Print and shaded views of the part. All mm, measured from the part's lowest x, y and z. A direction names the side the tool comes from. Round coordinates to 2 decimals unless told otherwise and drop trailing zeros. Write each loop counter-clockwise with the first axis right and the second up, starting at its lowest first coordinate (ties: lowest second). Pieces come first, ordered by that corner, then holes.
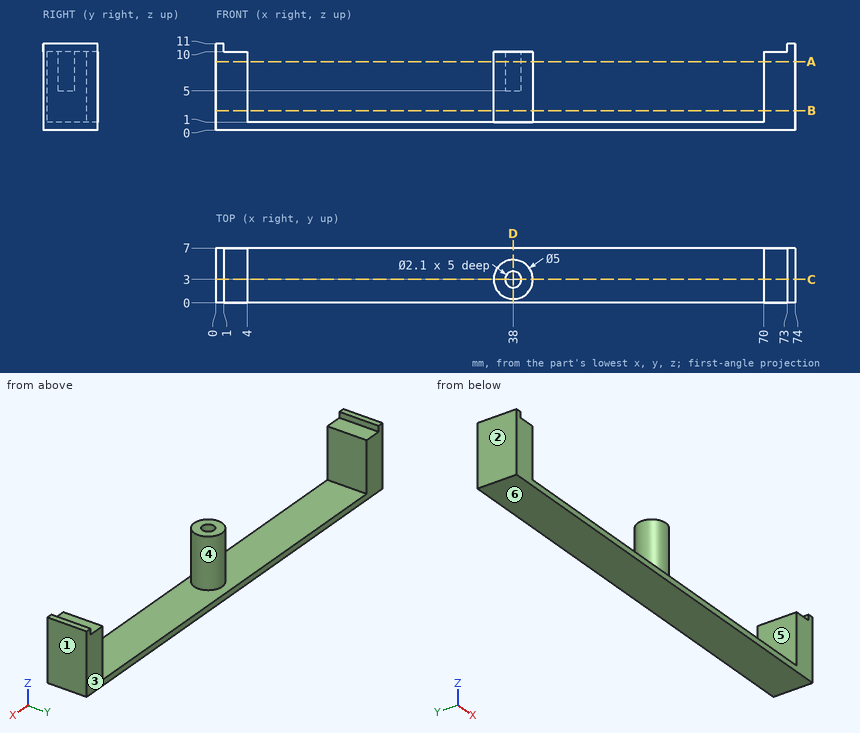
1) Slice it at A-A (z = 8.75). Write the cut outline in (x, y), plus the area to 3 significant figures.
Results:
outline: (0, 0) - (4, 0) - (4, 7) - (0, 7) - close; circle Ø5 at (38, 3); (70, 0) - (74, 0) - (74, 7) - (70, 7) - close; hole circle Ø2.1 at (38, 3)
area: 72.2 mm2
2) Slice it at C-C (y = 3). Write the cut outline in (x, z).
Results:
outline: (0, 0) - (74, 0) - (74, 11) - (73, 11) - (73, 10) - (70, 10) - (70, 1) - (40.5, 1) - (40.5, 10) - (39.05, 10) - (39.05, 5) - (36.95, 5) - (36.95, 10) - (35.5, 10) - (35.5, 1) - (4, 1) - (4, 10) - (1, 10) - (1, 11) - (0, 11) - close
3) Wall check: L1, parallel to X at y = 3, z = 8.25; L2, parallel to X at y = 6.5, z = 3.75; L3, parallel to X at y = 6.5, z = 10.5. Give the ranges that are in metal, low to high.
Results:
L1: x = 0 to 4, 35.5 to 36.95, 39.05 to 40.5, 70 to 74
L2: x = 0 to 4, 70 to 74
L3: x = 0 to 1, 73 to 74
4) Which spindle directions (+Z, -Z, +X, -X, +Y, -Y) get a long thin tool onto all of the face, cutting with end or side? Do the marked faces 5 and 6. Say none if no direction does.
Results:
face 5: +Z, +Y, -Y
face 6: -Z, +X, -X, +Y, -Y
5) Slice it at D-D (x = 38). Write the cut outline in (y, z).
Results:
outline: (0, 0) - (7, 0) - (7, 1) - (5.5, 1) - (5.5, 10) - (4.05, 10) - (4.05, 5) - (1.95, 5) - (1.95, 10) - (0.5, 10) - (0.5, 1) - (0, 1) - close
6) Slice it at B-B (z = 2.5). Write the cut outline in (x, y).
Results:
outline: (0, 0) - (4, 0) - (4, 7) - (0, 7) - close; circle Ø5 at (38, 3); (70, 0) - (74, 0) - (74, 7) - (70, 7) - close
7) Pin check, flat tips, straight feed: pin 1 Ø1.5 at (x, z) = (39, 7) entering from +Y; pin 2 Ø1 at (x, y) = (54.5, 5) entering from +Z; pin 3 Ø1.7 at (x, y) = (38, 3) entering from +Z. Stop position of each tip, or through.
Results:
pin 1: stops at y = 5.49
pin 2: stops at z = 1
pin 3: stops at z = 5
8) Mould opens along X. For the marked faces 1, 2, 3 and 4 say: released by +X, released by -X, zero draft, split by the parting line, or undercut.
Results:
face 1: released by +X
face 2: released by -X
face 3: zero draft
face 4: undercut
